Job drawing, mm, ordinate dimensions from the low corner. One solid piece. A direction names the side the tool comes from. Round coordinates to 2 decimals unless told otherwise and drop trailing zeros. Write each loop counter-clockwise with the first axis right and the second up, starting at its lowest first coordinate (ties: lowest second). Pieces come first, ordered by that corner, then holes.
1) Saw through at D-D (z = 8). Write the cut outline in (x, y), plus the area to 3 significant figures.
2) Which spindle directions (+Z, -Z, +X, -X, +Y, -Y) get a long thin tool onto all of the face, cutting with end or side? Do the marked faces 1, 2 and 3. Say none if no direction does.
3) Saw through at A-A (y = 45). Write the cut outline in (x, z), plus the area to 3 significant figures.
4) Pull direction X, two halves, no side cores. Call the marked faces 4, 5 and 6: +X half, -X half, draft (parallel to the pull), parting line (faces both ways), or undercut.
5) Saw through at B-B (x = 41.5). Write the cut outline in (y, z).
6) Flat gauge pins, fed straight in: pin 1 (10 mm diameter, centred on x = 52.5, z = 14.5, fed in from -Y) (3 decimals); pin 2 (8 mm diameter, centred on x = 10.5, y = 45, fed in from +Z); pin 3 (2 mm diameter, centred on x = 23.5, y = 23, fed in from -Z); pin 4 (12 mm diameter, centred on x = 35, y = 22, fed in from +Z). Where does each tip first touch, or does it go through?
7) Saw through at C-C (z = 26). Write the cut outline in (x, y).
8) Wall check: probe 1 along X at (y, z) = (44, 24); probe 2 along X at (y, z) = (10.5, 8); probe 3 along Y at (x, z) = (56.5, 39). Give the ranges that are in metal, low to high.
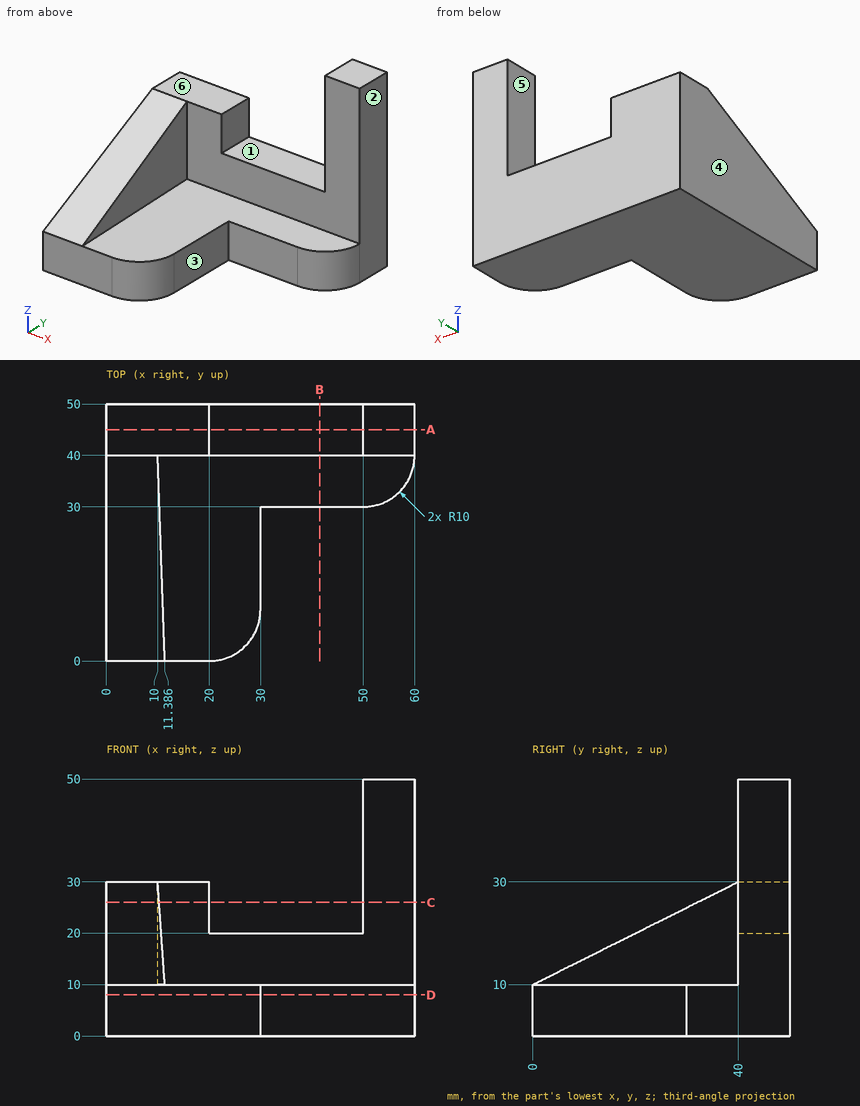
Evaluation:
1. outline: (0, 0) - (20, 0) arc R10 ccw to (30, 10) - (30, 30) - (50, 30) arc R10 ccw to (60, 40) - (60, 50) - (0, 50) - close
1. area: 2,060 mm2
2. face 1: +Z, +Y, -Y
2. face 2: +Z, -Z, +X, +Y, -Y
2. face 3: +Z, -Z, +X, -Y
3. outline: (0, 0) - (60, 0) - (60, 50) - (50, 50) - (50, 20) - (20, 20) - (20, 30) - (0, 30) - close
3. area: 1,700 mm2
4. face 4: -X half
4. face 5: undercut
4. face 6: draft
5. outline: (30, 0) - (50, 0) - (50, 20) - (40, 20) - (40, 10) - (30, 10) - close
6. pin 1: stops at y = 30.005
6. pin 2: stops at z = 30
6. pin 3: stops at z = 0
6. pin 4: stops at z = 10
7. outline: (0, 32) - (10.28, 32) - (10, 40) - (20, 40) - (20, 50) - (0, 50) - close; (50, 40) - (60, 40) - (60, 50) - (50, 50) - close
8. probe 1: x = 0 to 20, 50 to 60
8. probe 2: x = 0 to 30
8. probe 3: y = 40 to 50
